The model under review builds one solid part; all positions refer to its coordinate system, in mm. Face numbers are marked on the shaded views. Give positions to 0.01 mm unless a question says otherwise; leave off trailing zeros. Order: outer loops, then holes, each group sorted by start corner. A loop starts at its lowest first (then second) coordinate and runs counter-clockwise, first axis right, second up. Notation, with made-up numbers: M -30.75,47 L -26.75,47 A6 cw -26.75,57 Z; hole C 24,79.5 d3. An arc over 180 degrees is marked long. One line per question, with ' | ' between items. Start each with the question number.
1. Wall thickness on L1, parallel to Y at x = 0, z = 32; L2, parallel to X at y = -0.5, z = 30; L3, parallel to Z at x = 7, y = 3: over which ranges is each line inside the solid? List them lowest first.
2. We need section C-C on z = 47.5. Write out the cut boundary in (x, y), then the cut area to 3 significant figures.
3. The part is to be moulded in two halves that separate along X. For the marked faces 1, 2 and 3, say which applies: +X half, -X half, draft (parallel to the pull), parting line (faces both ways), or undercut.
4. We need section D-D on z = 36. Write out the cut boundary in (x, y).
5. We need section A-A on y = 0. Write out the cut boundary in (x, z).
6. Insertion check: P1, Ø1, axis at x = -9, y = 9.5, coming from the -Z side; P2, Ø8, axis at x = -9.5, y = -9, coming from the -Z side; P3, Ø3, axis at x = -10.5, z = 42.5, coming from the -Y side; P4, Ø10, axis at y = -10, z = 43, coming from the -X side. Each pin has a flat end and moves straight along its axis. Give the tip position at first contact, or say it passes through.
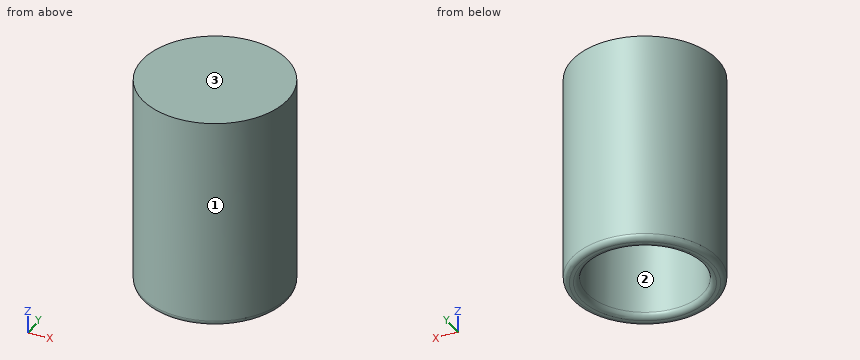
```python
from build123d import *

# Parameters (mm, degrees)
F0_R     = 18.3671775814
F0_R_2   = 14.6879268772
F1_DEPTH = 53.8542717695
F2_DEPTH = 46.8754135072
F3_R     = 1.3703832561


with BuildPart() as f1:
    # F0 (on Top) → F1 (new body)
    with BuildSketch(Plane.XY):
        Circle(F0_R)
        Circle(F0_R_2, mode=Mode.SUBTRACT)
        Circle(F0_R_2)
    extrude(amount=F1_DEPTH)

    # F0 (on Top) → F2 (cut)
    with BuildSketch(Plane.XY):
        Circle(F0_R_2)
    extrude(amount=F2_DEPTH, mode=Mode.SUBTRACT)

    # F3
    f3_edges = [f1.edges().sort_by_distance(p)[0] for p in [
        (-14.687927, 0, 0),
        (-18.367178, 0, 0),
    ]]
    fillet(f3_edges, radius=F3_R)


solid = f1.part
```
Entries:
1) L1: y = -18.37 to -14.69, 14.69 to 18.37 | L2: x = -18.36 to -14.68, 14.68 to 18.36 | L3: z = 46.88 to 53.85
2) outline: C 0,0 d36.73 | area: 1,060 mm^2
3) face 1: parting line | face 2: undercut | face 3: draft
4) outline: C 0,0 d36.73; hole C 0,0 d29.38
5) outline: M -18.37,1.37 A1.37 ccw -17,0 L -16.06,0 A1.37 ccw -14.69,1.37 L -14.69,46.88 L 14.69,46.88 L 14.69,1.37 A1.37 ccw 16.06,0 L 17,0 A1.37 ccw 18.37,1.37 L 18.37,53.85 L -18.37,53.85 Z
6) P1: stops at z = 46.88 | P2: stops at z = 0 | P3: stops at y = -16.01 | P4: stops at x = -17.67
